from build123d import *

# Parameters (mm, degrees)
SKETCH1_R           = 12
BOSS_EXTRUDE1_DEPTH = 7


with BuildPart() as part:
    # Sketch1 → Boss-Extrude1 (new body)
    with BuildSketch(Plane.XY):
        with BuildLine():
            Line((6.453651746, 28.272785132), (4.75543091, 25.561413828))
            ThreePointArc((4.75543091, 25.561413828), (3.133953687, 25.810430727), (1.5, 25.956694705))
            Line((1.5, 25.956694705), (0.5, 28.995689335))
            Line((0.5, 28.995689335), (-0.5, 28.995689335))
            Line((-0.5, 28.995689335), (-1.5, 25.956694705))
            ThreePointArc((-1.5, 25.956694705), (-3.133953687, 25.810430727), (-4.75543091, 25.561413828))
            Line((-4.75543091, 25.561413828), (-6.453651746, 28.272785132))
            Line((-6.453651746, 28.272785132), (-7.424593563, 28.033469468))
            Line((-7.424593563, 28.033469468), (-7.668256362, 24.843466835))
            ThreePointArc((-7.668256362, 24.843466835), (-9.219727063, 24.31042231), (-10.734493461, 23.680596491))
            Line((-10.734493461, 23.680596491), (-13.03224071, 25.906769425))
            Line((-13.03224071, 25.906769425), (-13.917696736, 25.442046253))
            Line((-13.917696736, 25.442046253), (-13.390861537, 22.286426974))
            ThreePointArc((-13.390861537, 22.286426974), (-14.769683415, 21.397580513), (-16.08970627, 20.423548961))
            Line((-16.08970627, 20.423548961), (-18.853443215, 22.035146447))
            Line((-18.853443215, 22.035146447), (-19.601953963, 21.372023789))
            Line((-19.601953963, 21.372023789), (-18.335238514, 18.434180986))
            ThreePointArc((-18.335238514, 18.434180986), (-19.461279452, 17.241189114), (-20.509843834, 15.979559002))
            Line((-20.509843834, 15.979559002), (-23.57895213, 16.882920851))
            Line((-23.57895213, 16.882920851), (-24.147016876, 16.059936985))
            Line((-24.147016876, 16.059936985), (-22.214038074, 13.510607405))
            ThreePointArc((-22.214038074, 13.510607405), (-23.021856667, 12.082802473), (-23.738023825, 10.606895158))
            Line((-23.738023825, 10.606895158), (-26.934138052, 10.749521263))
            Line((-26.934138052, 10.749521263), (-27.288742939, 9.81450502))
            Line((-27.288742939, 9.81450502), (-24.801838486, 7.80184643))
            ThreePointArc((-24.801838486, 7.80184643), (-25.244487253, 6.222207271), (-25.586636155, 4.617797121))
            Line((-25.586636155, 4.617797121), (-28.724009773, 3.991398571))
            Line((-28.724009773, 3.991398571), (-28.844546453, 2.998689697))
            Line((-28.844546453, 2.998689697), (-25.948246196, 1.639670499))
            ThreePointArc((-25.948246196, 1.639670499), (-26, 0), (-25.948246196, -1.639670499))
            Line((-25.948246196, -1.639670499), (-28.844546453, -2.998689697))
            Line((-28.844546453, -2.998689697), (-28.724009773, -3.991398571))
            Line((-28.724009773, -3.991398571), (-25.586636155, -4.617797121))
            ThreePointArc((-25.586636155, -4.617797121), (-25.244487253, -6.222207271), (-24.801838486, -7.80184643))
            Line((-24.801838486, -7.80184643), (-27.288742939, -9.81450502))
            Line((-27.288742939, -9.81450502), (-26.934138052, -10.749521263))
            Line((-26.934138052, -10.749521263), (-23.738023825, -10.606895158))
            ThreePointArc((-23.738023825, -10.606895158), (-23.021856667, -12.082802473), (-22.214038074, -13.510607405))
            Line((-22.214038074, -13.510607405), (-24.147016876, -16.059936985))
            Line((-24.147016876, -16.059936985), (-23.57895213, -16.882920851))
            Line((-23.57895213, -16.882920851), (-20.509843834, -15.979559002))
            ThreePointArc((-20.509843834, -15.979559002), (-19.461279452, -17.241189114), (-18.335238514, -18.434180986))
            Line((-18.335238514, -18.434180986), (-19.601953963, -21.372023789))
            Line((-19.601953963, -21.372023789), (-18.853443215, -22.035146447))
            Line((-18.853443215, -22.035146447), (-16.08970627, -20.423548961))
            ThreePointArc((-16.08970627, -20.423548961), (-14.769683415, -21.397580513), (-13.390861537, -22.286426974))
            Line((-13.390861537, -22.286426974), (-13.917696736, -25.442046253))
            Line((-13.917696736, -25.442046253), (-13.03224071, -25.906769425))
            Line((-13.03224071, -25.906769425), (-10.734493461, -23.680596491))
            ThreePointArc((-10.734493461, -23.680596491), (-9.219727063, -24.31042231), (-7.668256362, -24.843466835))
            Line((-7.668256362, -24.843466835), (-7.424593563, -28.033469468))
            Line((-7.424593563, -28.033469468), (-6.453651746, -28.272785132))
            Line((-6.453651746, -28.272785132), (-4.75543091, -25.561413828))
            ThreePointArc((-4.75543091, -25.561413828), (-3.133953687, -25.810430727), (-1.5, -25.956694705))
            Line((-1.5, -25.956694705), (-0.5, -28.995689335))
            Line((-0.5, -28.995689335), (0.5, -28.995689335))
            Line((0.5, -28.995689335), (1.5, -25.956694705))
            ThreePointArc((1.5, -25.956694705), (3.133953687, -25.810430727), (4.75543091, -25.561413828))
            Line((4.75543091, -25.561413828), (6.453651746, -28.272785132))
            Line((6.453651746, -28.272785132), (7.424593563, -28.033469468))
            Line((7.424593563, -28.033469468), (7.668256362, -24.843466835))
            ThreePointArc((7.668256362, -24.843466835), (9.219727063, -24.31042231), (10.734493461, -23.680596491))
            Line((10.734493461, -23.680596491), (13.03224071, -25.906769425))
            Line((13.03224071, -25.906769425), (13.917696736, -25.442046253))
            Line((13.917696736, -25.442046253), (13.390861537, -22.286426974))
            ThreePointArc((13.390861537, -22.286426974), (14.769683415, -21.397580513), (16.08970627, -20.423548961))
            Line((16.08970627, -20.423548961), (18.853443215, -22.035146447))
            Line((18.853443215, -22.035146447), (19.601953963, -21.372023789))
            Line((19.601953963, -21.372023789), (18.335238514, -18.434180986))
            ThreePointArc((18.335238514, -18.434180986), (19.461279452, -17.241189114), (20.509843834, -15.979559002))
            Line((20.509843834, -15.979559002), (23.57895213, -16.882920851))
            Line((23.57895213, -16.882920851), (24.147016876, -16.059936985))
            Line((24.147016876, -16.059936985), (22.214038074, -13.510607405))
            ThreePointArc((22.214038074, -13.510607405), (23.021856667, -12.082802473), (23.738023825, -10.606895158))
            Line((23.738023825, -10.606895158), (26.934138052, -10.749521263))
            Line((26.934138052, -10.749521263), (27.288742939, -9.81450502))
            Line((27.288742939, -9.81450502), (24.801838486, -7.80184643))
            ThreePointArc((24.801838486, -7.80184643), (25.244487253, -6.222207271), (25.586636155, -4.617797121))
            Line((25.586636155, -4.617797121), (28.724009773, -3.991398571))
            Line((28.724009773, -3.991398571), (28.844546453, -2.998689697))
            Line((28.844546453, -2.998689697), (25.948246196, -1.639670499))
            ThreePointArc((25.948246196, -1.639670499), (26, 0), (25.948246196, 1.639670499))
            Line((25.948246196, 1.639670499), (28.844546453, 2.998689697))
            Line((28.844546453, 2.998689697), (28.724009773, 3.991398571))
            Line((28.724009773, 3.991398571), (25.586636155, 4.617797121))
            ThreePointArc((25.586636155, 4.617797121), (25.244487253, 6.222207271), (24.801838486, 7.80184643))
            Line((24.801838486, 7.80184643), (27.288742939, 9.81450502))
            Line((27.288742939, 9.81450502), (26.934138052, 10.749521263))
            Line((26.934138052, 10.749521263), (23.738023825, 10.606895158))
            ThreePointArc((23.738023825, 10.606895158), (23.021856667, 12.082802473), (22.214038074, 13.510607405))
            Line((22.214038074, 13.510607405), (24.147016876, 16.059936985))
            Line((24.147016876, 16.059936985), (23.57895213, 16.882920851))
            Line((23.57895213, 16.882920851), (20.509843834, 15.979559002))
            ThreePointArc((20.509843834, 15.979559002), (19.461279452, 17.241189114), (18.335238514, 18.434180986))
            Line((18.335238514, 18.434180986), (19.601953963, 21.372023789))
            Line((19.601953963, 21.372023789), (18.853443215, 22.035146447))
            Line((18.853443215, 22.035146447), (16.08970627, 20.423548961))
            ThreePointArc((16.08970627, 20.423548961), (14.769683415, 21.397580513), (13.390861537, 22.286426974))
            Line((13.390861537, 22.286426974), (13.917696736, 25.442046253))
            Line((13.917696736, 25.442046253), (13.03224071, 25.906769425))
            Line((13.03224071, 25.906769425), (10.734493461, 23.680596491))
            ThreePointArc((10.734493461, 23.680596491), (9.219727063, 24.31042231), (7.668256362, 24.843466835))
            Line((7.668256362, 24.843466835), (7.424593563, 28.033469468))
            Line((7.424593563, 28.033469468), (6.453651746, 28.272785132))
        make_face()
        Circle(SKETCH1_R, mode=Mode.SUBTRACT)
    extrude(amount=BOSS_EXTRUDE1_DEPTH)


solid = part.part
Read the model definition and answer for the solid it produces. Units are mm, in the model's axes. A direction names the side the tool comes from. Round coordinates to 2 decimals unless told otherwise and drop trailing zeros. Write each loop counter-clockwise with the first axis right and the second up, starting at its lowest first coordinate (ties: lowest second). Pieces come first, ordered by that corner, then holes.
1. The part is cut by section B-B, the plane x = -9.5. Determine the outline of the cut face in (y, z).
2. The part is cut by section C-C, the plane x = 17. Determine the outline of the cut face in (y, z).
3. The part is cut by section A-A, the plane y = 0. Determine the outline of the cut face in (x, z).
4. Determine the mould class of faces 4 (the face through (1.01, 27.45, 3.45)), 5 (the face through (-25.25, -6.2, 3.45)), 6 (the face through (13.65, 23.84, 3.45)) for opening direction X: pulls with the +X half, pulls with the -X half, needs draft (parallel to the pull), parting line crosses it, or undercut.
5. Straight lines are drawn through the part: L1, parallel to Y at x = 24, z = 6.5; L2, parallel to Y at x = 0, z = 3.75; L3, parallel to X at y = -23, z = 5.25. For each, find the intervals that lie inside material, in ascending order.
6. Which of the six approach directions +Z, -Z, +X, -X, +Y, -Y give full straight-line access (tool end or side, diameter ignored) to faces 1 (the face through (27.38, 2.31, 3.45)), 2 (the face through (-14.75, 21.41, 3.45)), 3 (the face through (3.157, 25.808, 3.451))?
7. Given pin 1 Ø1 at (x, z) = (3, 3) entering from -Y; pin 2 Ø3 at (x, z) = (-5, 1) entering from +Y; pin 3 Ø1.5 at (x, y) = (15, -16) entering from -Z; pin 4 Ø3 at (y, z) = (-21, 1.5) entering from +X, each flat-ended and moving along its own axis, determine where each tip first touches the part or whether it passes through.
Values:
1. outline: (-24.2, 0) - (-7.33, 0) - (-7.33, 7) - (-24.2, 7) - close; (7.33, 0) - (24.2, 0) - (24.2, 7) - (7.33, 7) - close
2. outline: (-20.95, 0) - (20.95, 0) - (20.95, 7) - (-20.95, 7) - close
3. outline: (-26, 0) - (-12, 0) - (-12, 7) - (-26, 7) - close; (12, 0) - (26, 0) - (26, 7) - (12, 7) - close
4. face 4: undercut
4. face 5: pulls with the -X half
4. face 6: pulls with the +X half
5. L1: y = -16.27 to -15.87, -10.62 to 10.62, 15.87 to 16.27
5. L2: y = -29 to -12, 12 to 29
5. L3: x = -13.51 to 13.51
6. face 1: +Z, -Z, +X
6. face 2: +Z, -Z
6. face 3: +Z, -Z, +Y
7. pin 1: stops at y = -25.88
7. pin 2: stops at y = 28.27
7. pin 3: stops at z = 0
7. pin 4: stops at x = 19.6
